```python
from build123d import *

# Parameters (mm, degrees)
BOSS_EXTRUDE1_DEPTH = 35
CUT_EXTRUDE1_DEPTH  = 18
SKETCH3_R           = 1.25
CUT_EXTRUDE2_DEPTH  = 51.249378106
SKETCH5_R           = 0.518350726
CUT_EXTRUDE5_DEPTH  = 30
FILLET2_R           = 0.5
SKETCH7_R           = 2.25
CUT_EXTRUDE6_DEPTH  = 3
SKETCH8_R           = 2
CUT_EXTRUDE7_DEPTH  = 2.5
CUT_EXTRUDE8_START  = -2.5
SKETCH9_R           = 2
CUT_EXTRUDE8_DEPTH  = 2.5


with BuildPart() as part:
    # Sketch1 → Boss-Extrude1 (new, symmetric)
    with BuildSketch(Plane.XY):
        Polygon((-20, 5), (-20, 10), (-30, 5), align=None)
        Polygon((20, 10), (-20, 10), (-20, 5), (-20, -10), (20, -10), (20, 5), align=None)
        Polygon((30, 5), (20, 10), (20, 5), align=None)
    extrude(amount=BOSS_EXTRUDE1_DEPTH, both=True)

    # Sketch2 → Cut-Extrude1 (cut)
    with BuildSketch(Plane(origin=(0, 10, 0), x_dir=(1, 0, 0), z_dir=(0, 1, 0))):
        Polygon((-17.5, -13.5), (-17.5, -32.5), (17.5, -32.5), (17.5, -13.5), (12.7, -13.5), (12.7, 13.5), (17.5, 13.5), (17.5, 32.5), (-17.5, 32.5), (-17.5, 13.5), (-12.7, 13.5), (-12.7, -13.5), align=None)
    extrude(amount=-CUT_EXTRUDE1_DEPTH, mode=Mode.SUBTRACT)

    # Sketch3 → Cut-Extrude2 (cut, through all)
    with BuildSketch(Plane(origin=(0, 10, 0), x_dir=(1, 0, 0), z_dir=(0, 1, 0))):
        with Locations(Location((-24, 25, 0), (0, 0, 270))):
            Circle(SKETCH3_R)
        with Locations(Location((-24, -25, 0), (0, 0, 270))):
            Circle(SKETCH3_R)
        with Locations((24, 25)):
            Circle(SKETCH3_R)
        with Locations((24, -25)):
            Circle(SKETCH3_R)
    extrude(amount=-CUT_EXTRUDE2_DEPTH, mode=Mode.SUBTRACT)

    # Sketch5 → Cut-Extrude5 (cut, symmetric)
    with BuildSketch(Plane(origin=(0, 0, 0), x_dir=(-1, 0, 0), z_dir=(0, 0, -1))):
        with Locations((-13.9, 0)):
            Circle(SKETCH5_R)
        with Locations((13.9, 0)):
            Circle(SKETCH5_R)
    extrude(amount=CUT_EXTRUDE5_DEPTH, both=True, mode=Mode.SUBTRACT)

    # Fillet2
    fillet2_edges = [part.edges().sort_by_distance(p)[0] for p in [
        (-30, 5, 0),
        (30, 5, 0),
    ]]
    fillet(fillet2_edges, radius=FILLET2_R)

    # Sketch7 → Cut-Extrude6 (cut)
    with BuildSketch(Plane(origin=(0, 10, 0), x_dir=(1, 0, 0), z_dir=(0, 1, 0))):
        with Locations((-24, 25)):
            Circle(SKETCH7_R)
        with Locations((24, 25)):
            Circle(SKETCH7_R)
        with Locations((-24, -25)):
            Circle(SKETCH7_R)
        with Locations((24, -25)):
            Circle(SKETCH7_R)
    extrude(amount=-CUT_EXTRUDE6_DEPTH, mode=Mode.SUBTRACT)

    # Sketch8 → Cut-Extrude7 (cut)
    with BuildSketch(Plane.XY.offset(35)):
        with Locations((-13.9, 0)):
            Circle(SKETCH8_R)
        with Locations((13.9, 0)):
            Circle(SKETCH8_R)
    extrude(amount=-CUT_EXTRUDE7_DEPTH, mode=Mode.SUBTRACT)

    # Sketch9 → Cut-Extrude8 (cut)
    with BuildSketch(Plane(origin=(0, 0, -35), x_dir=(-1, 0, 0), z_dir=(0, 0, -1)).offset(CUT_EXTRUDE8_START)):
        with Locations(Location((13.9, 0, 0), (0, 0, 180))):
            Circle(SKETCH9_R)
        with Locations(Location((-13.9, 0, 0), (0, 0, 180))):
            Circle(SKETCH9_R)
    extrude(amount=CUT_EXTRUDE8_DEPTH, mode=Mode.SUBTRACT)


solid = part.part
```
Design review of the part built by this model. Coordinates are the model's own, in mm. A direction names the side the tool comes from. Coordinates: 2 decimals unless noted, no trailing zeros. Order: outer loops, then holes, each group sorted by start corner. A loop starts at its lowest first (then second) coordinate and runs counter-clockwise, first axis right, second up. Notation, with made-up numbers: (1.5, 43) -> (5.5, 43) arc R15 ccw to (5.5, 57) -> close; hole circle Ø1 at (51.25, 10). An arc over 180 degrees is marked (long way). One line per item, written item: value. Start each with the question number.
Q1. Take a section at B-B, the plane z = -7. State the section outline as (x, y) points.
Q2. Take a section at A-A, the plane x = -24. State the section outline as (y, z) points.
Q3. Mouldability with a two-part tool opening along Z and no side actions: class faces 1 (the cylindrical face through (-24.479, 6.014, 26.155)), 2 (the flat face through (0, 0, -35)), 3 (the flat face through (20, -3, 0)), 4 (the flat face through (0, 0, 35)) as pulls with the +Z half, pulls with the -Z half, needs draft (parallel to the pull), parting line crosses it, or undercut.
Q4. Insertion check: pin 1 Ø7 at (x, z) = (-24, -25) entering from -Y; pin 2 Ø4.5 at (y, z) = (-6, -14.5) entering from -X; pin 3 Ø3.5 at (x, z) = (-24.5, -24.5) entering from +Y; pin 4 Ø2 at (x, z) = (-24, 25) entering from +Y. Each pin has a flat end and moves straight along its axis. Give the tip position at first contact, or say it passes through.
Q5. For probe 1 along X at (y, z) = (5.5, -25); probe 2 along Z at (x, y) = (24, 5.5); probe 3 along X at (y, z) = (3, -18), list the stretches that pass through material, from the lowest coordinate up.
Q6. Tool access review of faces 5 (the flat face through (-20, -2, 0)), 6 (the flat face through (-15, 1, 13.5)), 7 (the flat face through (24, 5, 0)), 8 (the cylindrical face through (15.747, -0.766, 33.768)), 9 (the cylindrical face through (25.155, 6.014, 25.479)): name each direction out of +Z, -Z, +X, -X, +Y, -Y from which nothing blocks a thin tool from reaching the whole face with its end or side.
Q7. Take a section at C-C, the plane z = -25. State the section outline as (x, y) points (3 decimals).
Q8. Take a section at D-D, the plane x = -5.5. State the section outline as (y, z) points, then the cut area to 3 significant figures.
Values follow:
1. outline: (-28.11, 5.95) arc R0.5 ccw to (-27.88, 5) -> (-20, 5) -> (-20, -10) -> (20, -10) -> (20, 5) -> (27.88, 5) arc R0.5 ccw to (28.11, 5.95) -> (20, 10) -> (12.7, 10) -> (12.7, -8) -> (-12.7, -8) -> (-12.7, 10) -> (-20, 10) -> close; hole circle Ø1.04 at (-13.9, 0); hole circle Ø1.04 at (13.9, 0)
2. outline: (5, -35) -> (8, -35) -> (8, -27.25) -> (7, -27.25) -> (7, -26.25) -> (5, -26.25) -> close; (5, -23.75) -> (7, -23.75) -> (7, -22.75) -> (8, -22.75) -> (8, 22.75) -> (7, 22.75) -> (7, 23.75) -> (5, 23.75) -> close; (5, 26.25) -> (7, 26.25) -> (7, 27.25) -> (8, 27.25) -> (8, 35) -> (5, 35) -> close
3. face 1: undercut
3. face 2: pulls with the -Z half
3. face 3: needs draft
3. face 4: pulls with the +Z half
4. pin 1: stops at y = 5
4. pin 2: stops at x = -20
4. pin 3: stops at y = 7.87
4. pin 4: passes through
5. probe 1: x = -28.38 to -25.25, -22.75 to -17.5, 17.5 to 22.75, 25.25 to 28.38
5. probe 2: z = -35 to -26.25, -23.75 to 23.75, 26.25 to 35
5. probe 3: x = -20 to -17.5, 17.5 to 20
6. face 5: +Z, -Z, -X, -Y
6. face 6: +Y
6. face 7: +Z, -Z, +X, -Y
6. face 8: +Z
6. face 9: +Y, -Y
7. outline: (-28.106, 5.947) arc R0.5 ccw to (-27.882, 5) -> (-25.25, 5) -> (-25.25, 7) -> (-26, 7) -> close; (-22.75, 5) -> (-20, 5) -> (-20, -10) -> (20, -10) -> (20, 5) -> (22.75, 5) -> (22.75, 7) -> (21.75, 7) -> (21.75, 9.125) -> (20, 10) -> (17.5, 10) -> (17.5, -8) -> (-17.5, -8) -> (-17.5, 10) -> (-20, 10) -> (-21.75, 9.125) -> (-21.75, 7) -> (-22.75, 7) -> close; (25.25, 5) -> (27.882, 5) arc R0.5 ccw to (28.106, 5.947) -> (26, 7) -> (25.25, 7) -> close
8. outline: (-10, -35) -> (10, -35) -> (10, -32.5) -> (-8, -32.5) -> (-8, 32.5) -> (10, 32.5) -> (10, 35) -> (-10, 35) -> close
8. area: 230 mm2
